The listing builds one solid part. Answer for the finished solid, in the listing's coordinates (mm). Face numbers are marked on the shaded views. A direction names the side the tool comes from. Coordinates: 2 decimals unless noted, no trailing zeros. Order: outer loops, then holes, each group sorted by start corner. A loop starts at its lowest first (then second) coordinate and runs counter-clockwise, first axis right, second up. Notation, with made-up numbers: (-40, -18) -> (-13, -18) arc R27 cw to (-13, 11) -> close; hole circle Ø3 at (-2, 74.25). An arc over 180 degrees is marked (long way). Write each question's results on one line, items separated by ' | '. Start each with the question number.
(1) A tool of negligible diameter and unlimited length cuts with its end or side. For the marked faces 5 and 6, from which of +Z, -Z, +X, -X, +Y, -Y can it reach the whole face along a straight path? Write none if from no direction.
(2) The part is cut by section D-D, the plane x = -9. Give the vertices of the cut face in (y, z), then the cut area to 3 significant figures.
(3) The part is cut by section B-B, the plane x = 3. Give the vertices of the cut face in (y, z).
(4) The part is cut by section A-A, the plane z = -15. Give the vertices of the cut face in (x, y) (3 decimals), then the cut area to 3 significant figures.
(5) A straight line is drawn through the part: L1, parallel to Z at x = 1, y = -3. Find the intervals that lie inside material, in ascending order.
(6) Determine the mould class of the marked faces 1, 2, 3 and 4 for opening direction X: +X half, -X half, draft (parallel to the pull), parting line (faces both ways), or undercut.
(7) Given pin 1 (12 mm diameter, centred on x = -10, z = 6, fed in from +Y), flat-ended and moving along its own axis, determine where the tip first touches the part or whether it passes through.
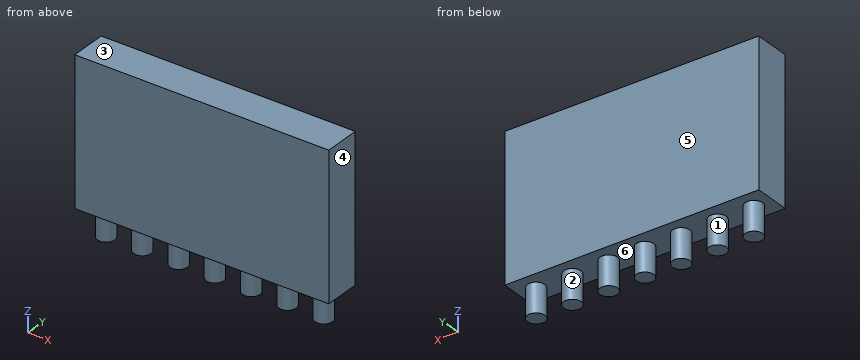
```python
from build123d import *

# Parameters (mm, degrees)
F0_W     = 50.8
F0_H     = 25.4
F1_DEPTH = 6.35
F2_R     = 1.524
F3_DEPTH = 5.08
F4_W     = 6.35
F4_H     = 61.243406
F5_DEPTH = 25.4


with BuildPart() as f1:
    # F0 (on Front) → F1 (new body)
    with BuildSketch(Plane.XZ):
        Rectangle(F0_W, F0_H)
    extrude(amount=F1_DEPTH)

    # F2 (on face) → F3 (join)
    with BuildSketch(Plane(origin=(0, 0, -12.7), x_dir=(1, 0, 0), z_dir=(0, 0, -1))):
        with BuildLine():
            ThreePointArc((-23.749, 3.175), (-22.225, 1.651), (-20.701, 3.175))
            ThreePointArc((-20.701, 3.175), (-22.225, 4.699), (-23.749, 3.175))
        make_face()
        with Locations((-15.875, 3.175)):
            Circle(F2_R)
        with Locations((-9.525, 3.175)):
            Circle(F2_R)
        with Locations((-3.175, 3.175)):
            Circle(F2_R)
        with Locations((3.175, 3.175)):
            Circle(F2_R)
        with Locations((9.525, 3.175)):
            Circle(F2_R)
        with Locations((15.875, 3.175)):
            Circle(F2_R)
        with Locations((22.225, 3.175)):
            Circle(F2_R)
    extrude(amount=F3_DEPTH)

    # F4 (on face) → F5 (cut)
    with BuildSketch(Plane.XZ.offset(6.35)):
        with Locations((22.225, -17.921703)):
            Rectangle(F4_W, F4_H)
    extrude(amount=-F5_DEPTH, mode=Mode.SUBTRACT)


solid = f1.part
```
Established:
1) face 5: +Z, -Z, +X, -X, +Y | face 6: -Z
2) outline: (-6.35, -12.7) -> (-4.61, -12.7) -> (-4.61, -17.78) -> (-1.74, -17.78) -> (-1.74, -12.7) -> (0, -12.7) -> (0, 12.7) -> (-6.35, 12.7) -> close | area: 176 mm^2
3) outline: (-6.35, -12.7) -> (-4.69, -12.7) -> (-4.69, -17.78) -> (-1.66, -17.78) -> (-1.66, -12.7) -> (0, -12.7) -> (0, 12.7) -> (-6.35, 12.7) -> close
4) outline: circle Ø3.048 at (-22.225, -3.175); circle Ø3.048 at (-15.875, -3.175); circle Ø3.048 at (-9.525, -3.175); circle Ø3.048 at (-3.175, -3.175); circle Ø3.048 at (3.175, -3.175); circle Ø3.048 at (9.525, -3.175); circle Ø3.048 at (15.875, -3.175) | area: 51.1 mm^2
5) L1: z = -12.7 to 12.7
6) face 1: undercut | face 2: undercut | face 3: draft | face 4: +X half
7) pin 1: stops at y = 0
